Autodesk Inventor part; units mm, degrees
ref_plane "YZ Plane" through (0, 0, 0) normal (1, 0, 0) x (0, 1, 0)
ref_plane "XZ Plane" through (0, 0, 0) normal (0, 1, 0) x (-1, 0, 0)
ref_plane "XY Plane" through (0, 0, 0) normal (0, 0, 1) x (1, 0, 0)
sketch "Skizze1" plane through (0, 0, 0) normal (0, 0, 1) x (1, 0, 0)
  line L0 (-240.4724, 39.0464) -> (579.5276, 39.0464)
  line L1 (579.5276, 39.0464) -> (579.5276, -160.9536)
  line L2 (579.5276, -160.9536) -> (-240.4724, -160.9536)
  line L3 (-240.4724, -160.9536) -> (-240.4724, 39.0464)
  point P0 (0, 0)
  dimension "d0" = 200
  dimension "d1" = 820
extrude "Extrusion1" add sketch "Skizze1" along normal blind 800
fillet "Rundung1" radius 410 2 edges at (-240.4724, -60.9536, 800) (579.5276, -60.9536, 800)
sketch "Skizze2" plane through (-240.4724, -160.9536, 0) normal (0, -1, 0) x (1, 0, 0)
  circle A0 centre (410, 390) radius 360
  line L0 (820, 0) -> (820, 390)
  line L1 (0, 0) -> (820, 0)
  point P0 (240.4724, 0)
  dimension "d5" = 720
  dimension "d6" = 410
  dimension "d7" = 390
extrude "Extrusion2" cut sketch "Skizze2" against normal up to surface (200 mm away)
properties part number "XPS-Hinten"
Can you work these out from the model? Positions are in its coordinate system, mm. Coordinates: 2 decimals unless noted, no trailing zeros. Order: outer loops, then holes, each group sorted by start corner. A loop starts at its lowest first (then second) coordinate and runs counter-clockwise, first axis right, second up. Notation, with made-up numbers: (-12, 89) - (24, 89) arc R19 cw to (24, 97) - close; hole circle Ø4 at (-0.75, -13.75). An arc over 180 degrees is marked (long way). Answer as a JSON object with one key per item and string values. Group by question number.
Q1. I need wall thicknesses on line 1 (X direction, y = -124, z = 171); line 2 (Z direction, x = 192.5, y = -147); line 3 (X direction, y = -2.5, z = 669). Which ranges of each line are inside material? Lowest first, please. Write a range as from..to.
Q2. Imagine slicing it at C-C (z = 331). Please give me the cut outline in (x, y), and give its area (3 significant figures).
Q3. Will these pins go through, and if not, where does the flat tip stop? P1, Ø2, axis at x = 301, y = -28.5, coming from the +Z side; P2, Ø1, axis at y = -57, z = 486.5, coming from the +X side; P3, Ø12, axis at x = 233.5, y = -72, coming from the +Z side.
Q4. We'd pull the mould along Z, two halves only. Please class faces 1 (the face through (91.49, -62.35, 38.56)), 2 (the face through (462.61, -62.35, 676.71)), 3 (the face through (579.528, -60, 192)): +Z half, -Z half, draft (parallel to the pull), parting line (faces both ways), or undercut.
Q5. Imagine slicing it at B-B (x = 273.5). Please give me the cut outline in (y, z).
Determined:
{
 "1": {"line 1": "x = -240.47..-116.2, 455.25..579.53", "line 2": "z = 0..30.73, 749.27..799.36", "line 3": "x = -130.9..-57.98, 397.03..469.96"},
 "2": {"outline": "(-240.47, -160.95) - (-185.6, -160.95) - (-185.6, 39.05) - (-240.47, 39.05) - close; (524.66, -160.95) - (579.53, -160.95) - (579.53, 39.05) - (524.66, 39.05) - close", "area": "21,900 mm2"},
 "3": {"P1": "stops at z = 778.69", "P2": "stops at x = 568.13", "P3": "stops at z = 795.88"},
 "4": {"face 1": "undercut", "face 2": "+Z half", "face 3": "draft"},
 "5": {"outline": "(-160.95, 0) - (39.05, 0) - (39.05, 45.34) - (-160.95, 45.34) - close; (-160.95, 734.66) - (39.05, 734.66) - (39.05, 786.6) - (-160.95, 786.6) - close"}
}
